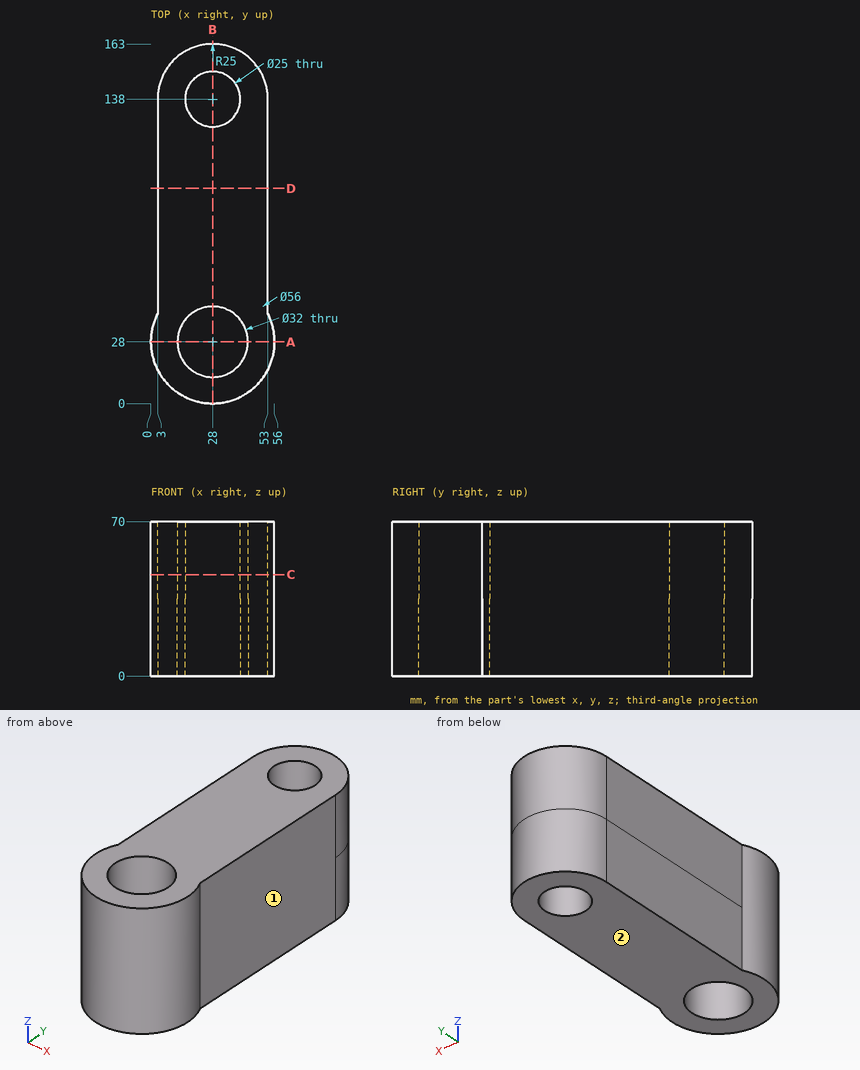
Can you work these out from the drawing? Everything is in mm from the part's minimum corner. A direction names the side the tool comes from. Round coordinates to 2 decimals unless told otherwise and drop trailing zeros. Loops run counter-clockwise (first coordinate to the right, second up) from the corner with the lowest first, then second, coordinate; pieces in that order, holes last. Notation, with made-up numbers: (15, 11) - (62, 11) arc R14 ccw to (62, 35) - close; hole circle Ø5 at (-39.75, 9). An arc over 180 degrees is marked (long way). Answer as CSV lines item,"result".
1. I want a section at C-C on z = 46. List the corners of the cut face in (x, y) for me.
Filled in:
outline,"(3, 40.61) arc R28 ccw (long way) to (53, 40.61) - (53, 138) arc R25 ccw to (3, 138) - close; hole circle Ø32 at (28, 28); hole circle Ø25 at (28, 138)"
2. I want a section at D-D on y = 97.5. List the corners of the cut face in (x, z) for me, then the cut area to 3 significant figures.
Filled in:
outline,"(3, 0) - (53, 0) - (53, 70) - (3, 70) - close"
area,"3,500 mm^2"
3. I want a section at B-B on x = 28. List the corners of the cut face in (y, z) for me.
Filled in:
outline,"(0, 0) - (12, 0) - (12, 70) - (0, 70) - close; (44, 0) - (125.5, 0) - (125.5, 70) - (44, 70) - close; (150.5, 0) - (163, 0) - (163, 70) - (150.5, 70) - close"
4. I want a section at A-A on y = 28. List the corners of the cut face in (x, z) for me.
Filled in:
outline,"(0, 0) - (12, 0) - (12, 70) - (0, 70) - close; (44, 0) - (56, 0) - (56, 70) - (44, 70) - close"
5. For pin 1 Ø12 at (x, z) = (48.5, 40.5) entering from -Y; pin 2 Ø8 at (y, z) = (53.5, 34) entering from +X; pin 3 Ø10 at (y, z) = (33, 19) entering from +X; pin 4 Ø12 at (x, y) = (23, 41.5) entering from -Z, each with a flat end and sliding along its axis, tell me the tip position at first contact or that it passes through.
Filled in:
pin 1,"stops at y = 4.05"
pin 2,"stops at x = 53"
pin 3,"stops at x = 56"
pin 4,"stops at z = 0"
6. Please list where these lines run through material, in increasing order: line 1 along Y through (x, z) = (28, 43); line 2 along X through (y, z) = (137.5, 8); line 3 along Y through (x, z) = (32, 57). Write a range as [from, to].
Filled in:
line 1,"y = [0, 12], [44, 125.5], [150.5, 163]"
line 2,"x = [3, 15.51], [40.49, 53]"
line 3,"y = [0.29, 12.51], [43.49, 126.16], [149.84, 162.68]"
7. On a 3-axis mill with a long thin cutter (end or side, diameter ignored), from which of +Z, -Z, +X, -X, +Y, -Y can I reach the whole of each face in a straight line? I mean the marked faces 1 and 2. Say none if no direction works.
Filled in:
face 1,"+Z, -Z, +X, +Y"
face 2,"-Z, +X, -X, +Y, -Y"
